```python
from build123d import *

# Parameters (mm, degrees)
SPUR_START             = -65.99548243
SPUR_GEAR_AM_OUTLINE_R = 2
SPUR_GEAR_AM_DEPTH     = 8.001
SKETCH1_R              = 2.4892
CUT_EXTRUDE1_DEPTH     = 38.916221237


# Read off the part's stored shape, not the designer's step: spur gear_am
with BuildPart() as part:
    # spur gear_am outline → spur gear_am (new body)
    with BuildSketch(Plane.YZ.offset(SPUR_START)):
        with BuildLine():
            ThreePointArc((15.314879055, 24.539540588), (15.391528072, 24.659938624), (15.465138567, 24.782218033))
            ThreePointArc((15.465138567, 24.782218033), (15.063480167, 25.38187856), (14.478147109, 25.804143203))
            ThreePointArc((14.478147109, 25.804143203), (14.600612124, 26.089561946), (14.70239475, 26.38299309))
            ThreePointArc((14.70239475, 26.38299309), (15.41943895, 26.300714095), (16.120256774, 26.473273058))
            ThreePointArc((16.120256774, 26.473273058), (16.148237066, 26.613229702), (16.172704392, 26.753843033))
            ThreePointArc((16.172704392, 26.753843033), (15.58154672, 27.167914071), (14.883200315, 27.350217435))
            ThreePointArc((14.883200315, 27.350217435), (14.894290398, 27.660601953), (14.883200315, 27.970986471))
            ThreePointArc((14.883200315, 27.970986471), (15.58154672, 28.153289835), (16.172704392, 28.567360874))
            ThreePointArc((16.172704392, 28.567360874), (16.148237066, 28.707974205), (16.120256774, 28.847930848))
            ThreePointArc((16.120256774, 28.847930848), (15.41943895, 29.020489811), (14.70239475, 28.938210816))
            ThreePointArc((14.70239475, 28.938210816), (14.600612124, 29.23164196), (14.478147109, 29.517060703))
            ThreePointArc((14.478147109, 29.517060703), (15.063480167, 29.939325346), (15.465138567, 30.538985873))
            ThreePointArc((15.465138567, 30.538985873), (15.391528072, 30.661265282), (15.314879055, 30.781663318))
            ThreePointArc((15.314879055, 30.781663318), (14.599050409, 30.68940516), (13.960149206, 30.35365604))
            ThreePointArc((13.960149206, 30.35365604), (13.759240179, 30.590504307), (13.541939811, 30.812409893))
            ThreePointArc((13.541939811, 30.812409893), (13.93520705, 31.417606636), (14.093119986, 32.121869174))
            ThreePointArc((14.093119986, 32.121869174), (13.980307826, 32.209300149), (13.865341959, 32.293879155))
            ThreePointArc((13.865341959, 32.293879155), (13.231179117, 31.949263852), (12.756708059, 31.405389388))
            ThreePointArc((12.756708059, 31.405389388), (12.483806507, 31.553667107), (12.201018405, 31.682089957))
            ThreePointArc((12.201018405, 31.682089957), (12.349106905, 32.388483625), (12.241947359, 33.102233616))
            ThreePointArc((12.241947359, 33.102233616), (12.105169441, 33.143008119), (11.967413502, 33.180345233))
            ThreePointArc((11.967413502, 33.180345233), (11.500563669, 32.629914991), (11.254602702, 31.951368441))
            ThreePointArc((11.254602702, 31.951368441), (10.946565493, 31.991049886), (10.636481757, 32.008645782))
            ThreePointArc((10.636481757, 32.008645782), (10.519391345, 32.720833997), (10.161631808, 33.347675549))
            ThreePointArc((10.161631808, 33.347675549), (10.019360749, 33.336286758), (9.87741944, 33.321339395))
            ThreePointArc((9.87741944, 33.321339395), (9.640933273, 32.639432869), (9.656700788, 31.917855705))
            ThreePointArc((9.656700788, 31.917855705), (9.355130054, 31.843581675), (9.059629211, 31.747974194))
            ThreePointArc((9.059629211, 31.747974194), (8.693173595, 32.369771991), (8.133131476, 32.82504668))
            ThreePointArc((8.133131476, 32.82504668), (8.00458177, 32.763032714), (7.877625051, 32.697819598))
            ThreePointArc((7.877625051, 32.697819598), (7.903441318, 31.976532042), (8.178807825, 31.309377259))
            ThreePointArc((8.178807825, 31.309377259), (7.924432364, 31.131178875), (7.68342344, 30.935280336))
            ThreePointArc((7.68342344, 30.935280336), (7.117094483, 31.382710477), (6.430406572, 31.604930933))
            ThreePointArc((6.430406572, 31.604930933), (6.33293957, 31.500667122), (6.23811365, 31.393995646))
            ThreePointArc((6.23811365, 31.393995646), (6.52274572, 30.730740941), (7.020521446, 30.208111489))
            ThreePointArc((7.020521446, 30.208111489), (6.847696075, 29.950055429), (6.69372866, 29.680323017))
            ThreePointArc((6.69372866, 29.680323017), (6.004012226, 29.892957582), (5.283419531, 29.852111701))
            ThreePointArc((5.283419531, 29.852111701), (5.23019869, 29.71967945), (5.180310335, 29.585956188))
            ThreePointArc((5.180310335, 29.585956188), (5.685317071, 29.070310558), (6.338274646, 28.76279044))
            ThreePointArc((6.338274646, 28.76279044), (6.270340387, 28.459728606), (6.224208635, 28.152591177))
            ThreePointArc((6.224208635, 28.152591177), (5.504254749, 28.10171269), (4.847077307, 27.803316934))
            ThreePointArc((4.847077307, 27.803316934), (4.845290398, 27.660601953), (4.847077307, 27.517886972))
            ThreePointArc((4.847077307, 27.517886972), (5.504254749, 27.219491216), (6.224208635, 27.168612729))
            ThreePointArc((6.224208635, 27.168612729), (6.270340387, 26.8614753), (6.338274646, 26.558413466))
            ThreePointArc((6.338274646, 26.558413466), (5.685317071, 26.250893348), (5.180310335, 25.735247718))
            ThreePointArc((5.180310335, 25.735247718), (5.23019869, 25.601524456), (5.283419531, 25.469092205))
            ThreePointArc((5.283419531, 25.469092205), (6.004012226, 25.428246324), (6.69372866, 25.640880889))
            ThreePointArc((6.69372866, 25.640880889), (6.847696075, 25.371148477), (7.020521446, 25.113092417))
            ThreePointArc((7.020521446, 25.113092417), (6.52274572, 24.590462965), (6.23811365, 23.927208261))
            ThreePointArc((6.23811365, 23.927208261), (6.33293957, 23.820536784), (6.430406572, 23.716272973))
            ThreePointArc((6.430406572, 23.716272973), (7.117094483, 23.938493429), (7.68342344, 24.38592357))
            ThreePointArc((7.68342344, 24.38592357), (7.924432364, 24.190025032), (8.178807825, 24.011826648))
            ThreePointArc((8.178807825, 24.011826648), (7.903441318, 23.344671864), (7.877625051, 22.623384308))
            ThreePointArc((7.877625051, 22.623384308), (8.00458177, 22.558171192), (8.133131476, 22.496157226))
            ThreePointArc((8.133131476, 22.496157226), (8.693173595, 22.951431915), (9.059629211, 23.573229712))
            ThreePointArc((9.059629211, 23.573229712), (9.355130054, 23.477622231), (9.656700788, 23.403348202))
            ThreePointArc((9.656700788, 23.403348202), (9.640933273, 22.681771038), (9.87741944, 21.999864511))
            ThreePointArc((9.87741944, 21.999864511), (10.019360749, 21.984917148), (10.161631808, 21.973528357))
            ThreePointArc((10.161631808, 21.973528357), (10.519391345, 22.600369909), (10.636481757, 23.312558124))
            ThreePointArc((10.636481757, 23.312558124), (10.946565493, 23.33015402), (11.254602702, 23.369835465))
            ThreePointArc((11.254602702, 23.369835465), (11.500563669, 22.691288915), (11.967413502, 22.140858673))
            ThreePointArc((11.967413502, 22.140858673), (12.105169441, 22.178195787), (12.241947359, 22.21897029))
            ThreePointArc((12.241947359, 22.21897029), (12.349106905, 22.932720281), (12.201018405, 23.639113949))
            ThreePointArc((12.201018405, 23.639113949), (12.483806507, 23.767536799), (12.756708059, 23.915814519))
            ThreePointArc((12.756708059, 23.915814519), (13.231179116, 23.371940054), (13.865341959, 23.027324751))
            ThreePointArc((13.865341959, 23.027324751), (13.980307825, 23.111903758), (14.093119986, 23.199334732))
            ThreePointArc((14.093119986, 23.199334732), (13.93520705, 23.90359727), (13.541939811, 24.508794013))
            ThreePointArc((13.541939811, 24.508794013), (13.759240179, 24.730699599), (13.960149206, 24.967547866))
            ThreePointArc((13.960149206, 24.967547866), (14.599050409, 24.631798746), (15.314879055, 24.539540588))
        make_face()
        with Locations((10.545290398, 27.660601953)):
            Circle(SPUR_GEAR_AM_OUTLINE_R, mode=Mode.SUBTRACT)
    extrude(amount=SPUR_GEAR_AM_DEPTH)

    # Sketch1 → Cut-Extrude1 (cut, through all)
    with BuildSketch(Plane(origin=(-57.99448243, 0, 0), x_dir=(0, 0, -1), z_dir=(1, 0, 0))):
        with Locations((-27.660601953, 10.545290398)):
            Circle(SKETCH1_R)
    extrude(amount=-CUT_EXTRUDE1_DEPTH, mode=Mode.SUBTRACT)


solid = part.part
```
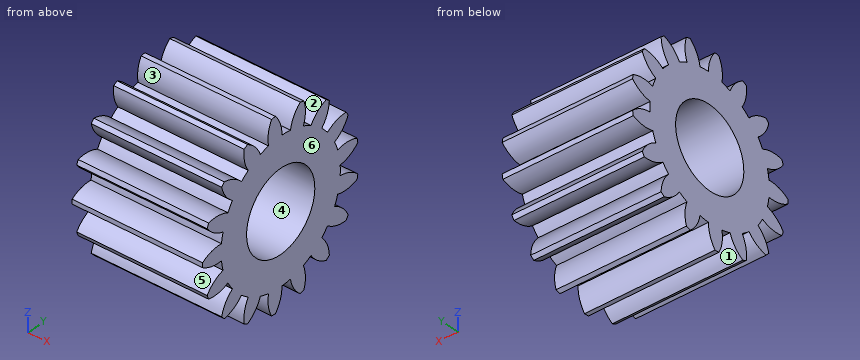
The model under review builds one solid part; all positions refer to its coordinate system, in mm. Face numbers are marked on the shaded views. A direction names the side the tool comes from. Coordinates: 2 decimals unless noted, no trailing zeros. Write each loop counter-clockwise with the first axis right and the second up, starting at its lowest first coordinate (ties: lowest second). Pieces come first, ordered by that corner, then holes. Notation, with made-up numbers: (36.25, -33) - (76.25, -33) arc R18 cw to (76.25, -12) - close; hole circle Ø7 at (19, -11.75). An arc over 180 degrees is marked (long way). Answer in a Markdown table with one row per item. Add a question column.
Q1. To check wall thickness, follow line 1 along Z through (x, y) = (-61.25, 15.25); line 2 along Z through (x, y) = (-60.5, 14.75); line 3 along Z through (x, y) = (-63.25, 11.5). State the ranges of each line that lie inside material, in increasing order. Write a range as from..to.
Q2. Consider section A-A on z = 26. Give the boundary of the cut face in (x, y), then the cut area to 3 significant figures.
Q3. Draft analysis for pull direction Y (two halves, no side actions). For the marked faces 4, 5 and 6, state which applies: +Y half, -Y half, draft (parallel to the pull), parting line (faces both ways), or undercut.
Q4. Clearance check with a flat-ended pin moving along its axis: pin 1 (1 mm diameter, centred on x = -64, y = 7, fed in from +Z). State where the tip first meets the part, or that it passes through.
Q5. For the marked faces 1, 2 and 3, list the 3-axis set-ups (+Z, -Z, +X, -X, +Y, -Y) from which the entire face can be reached by the end or side of a thin tool; tool diameter is ignored.
Answers below:
| question | item | result |
|---|---|---|
| 1 | line 1 | 24.54..25.16, 26.3..27.29, 28.03..29.02, 30.16..30.78 |
| 1 | line 2 | 24.59..25.65, 26.37..28.95, 29.67..30.73 |
| 1 | line 3 | 22.69..25.36, 29.96..32.63 |
| 2 | outline | (-66, 5.39) - (-57.99, 5.39) - (-57.99, 8.69) - (-66, 8.69) - close; (-66, 12.4) - (-57.99, 12.4) - (-57.99, 14.56) - (-66, 14.56) - close |
| 2 | area | 43.7 mm² |
| 3 | face 4 | undercut |
| 3 | face 5 | -Y half |
| 3 | face 6 | draft |
| 4 | pin 1 | z = 31.59 |
| 5 | face 1 | -Z, +X, -X |
| 5 | face 2 | +Z, +X, -X |
| 5 | face 3 | +X, -X |
